Source: three-view drawing plus pictorial views. Frame: mm from the lowest corner of the part. Give positions to 0.01 mm unless a question says otherwise; leave off trailing zeros. Loops run counter-clockwise (first coordinate to the right, second up) from the corner with the lowest first, then second, coordinate; pieces in that order, holes last.
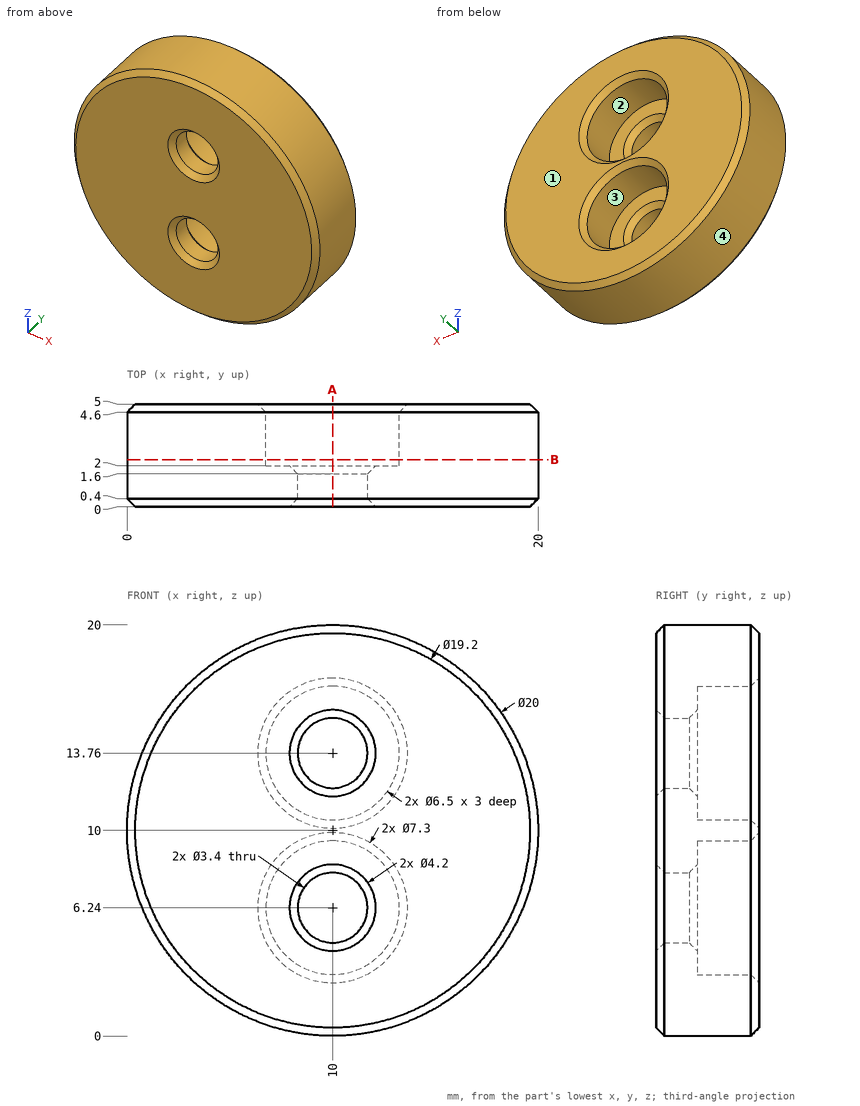
1) Ray query, probe 1 along Z at (x, y) = (10.25, 2.3); probe 2 along Z at (x, y) = (13, 3.5); probe 3 along X at (y, z) = (1.25, 6.24). Return the intervals inside material, ascending.
Checks:
probe 1: z = 0 to 3, 9.48 to 10.52, 17 to 20
probe 2: z = 0.46 to 4.99, 7.49 to 12.51, 15.01 to 19.54
probe 3: x = 0.73 to 8.3, 11.7 to 19.27
2) Cut plane A-A (x = 10). State how many separate pieces and enclosed holes the cut face has, and give its area (3 significant figures).
Checks:
separate pieces: 3
enclosed holes: 0
area: 46.1 mm2
3) Cut plane B-B (y = 2.3). Return loops of the section in (x, z), and give its area (3 significant figures).
Checks:
outline: circle Ø20 at (10, 10); hole circle Ø6.5 at (10, 6.24); hole circle Ø6.5 at (10, 13.76)
area: 248 mm2
4) Pull-direction query (X, two-part tool) for the marked faces 1, 2, 3 and 4; classes: released by +X, released by -X, zero draft, split by the parting line, or undercut.
Checks:
face 1: zero draft
face 2: undercut
face 3: undercut
face 4: split by the parting line
5) Contact query for flat-ended pins moving along their axis: P1, Ø6, axis at x = 10, z = 13.76, coming from the +Y side; P2, Ø4, axis at x = 10, z = 6.24, coming from the +Y side; P3, Ø1, axis at y = 2, z = 5, coming from the -X side; P4, Ø1.9, axis at x = 9.5, z = 13.5, coming from the +Y side. Output: stop coordinate, or through.
Checks:
P1: stops at y = 2
P2: stops at y = 1.9
P3: stops at x = 1.07
P4: passes through
